Part model, mm, in its own coordinate system. A direction names the side the tool comes from. Give positions to 0.01 mm unless a question says otherwise; leave off trailing zeros. Write each loop counter-clockwise with the first axis right and the second up, starting at its lowest first coordinate (ties: lowest second). Pieces come first, ordered by that corner, then holes. Notation, with made-up numbers: (-36.5, 70) - (-13.5, 70) arc R9 ccw to (-13.5, 74) - close; hole circle Ø9 at (35, 22.5). An arc over 180 degrees is marked (long way). Answer as a JSON object with one key per item and string values. Group by question number.
```python
from build123d import *

# Parameters (mm, degrees)
EXTRUDE_1_DEPTH = 1.68
SKETCH_2_R      = 14.75
EXTRUDE_3_DEPTH = 5


with BuildPart() as part:
    # 草图1 → 凸台-拉伸1 (new body)
    with BuildSketch(Plane(origin=(0, 0, 0), x_dir=(1, 0, 0), z_dir=(0, 1, 0))):
        with BuildLine():
            ThreePointArc((-21.5, 23.6), (-19.6254834, 28.1254834), (-15.1, 30))
            Line((-15.1, 30), (15.1, 30))
            ThreePointArc((15.1, 30), (19.6254834, 28.1254834), (21.5, 23.6))
            Line((21.5, 23.6), (21.5, -23.6))
            ThreePointArc((21.5, -23.6), (19.6254834, -28.1254834), (15.1, -30))
            Line((15.1, -30), (-15.1, -30))
            ThreePointArc((-15.1, -30), (-19.6254834, -28.1254834), (-21.5, -23.6))
            Line((-21.5, -23.6), (-21.5, 23.6))
        make_face()
        with BuildLine():
            ThreePointArc((-18.2, -23.95), (-15, -27.15), (-11.8, -23.95))
            Line((-11.8, -23.95), (-11.8, -21.05))
            ThreePointArc((-11.8, -21.05), (-15, -17.85), (-18.2, -21.05))
            Line((-18.2, -21.05), (-18.2, -23.95))
        make_face(mode=Mode.SUBTRACT)
        with BuildLine():
            ThreePointArc((18.2, -21.05), (15, -17.85), (11.8, -21.05))
            Line((11.8, -21.05), (11.8, -23.95))
            ThreePointArc((11.8, -23.95), (15, -27.15), (18.2, -23.95))
            Line((18.2, -23.95), (18.2, -21.05))
        make_face(mode=Mode.SUBTRACT)
        with BuildLine():
            ThreePointArc((18.2, 23.95), (15, 27.15), (11.8, 23.95))
            Line((11.8, 23.95), (11.8, 21.05))
            ThreePointArc((11.8, 21.05), (15, 17.85), (18.2, 21.05))
            Line((18.2, 21.05), (18.2, 23.95))
        make_face(mode=Mode.SUBTRACT)
        with BuildLine():
            ThreePointArc((-18.2, 21.05), (-15, 17.85), (-11.8, 21.05))
            Line((-11.8, 21.05), (-11.8, 23.95))
            ThreePointArc((-11.8, 23.95), (-15, 27.15), (-18.2, 23.95))
            Line((-18.2, 23.95), (-18.2, 21.05))
        make_face(mode=Mode.SUBTRACT)
    extrude(amount=EXTRUDE_1_DEPTH)

    # 草图2 → 凸台-拉伸3 (add)
    with BuildSketch(Plane(origin=(0, 1.68, 0), x_dir=(1, 0, 0), z_dir=(0, 1, 0))):
        Circle(SKETCH_2_R)
    extrude(amount=EXTRUDE_3_DEPTH)


solid = part.part
```
1) Saw through at D-D (z = 0). List the corners of the cut face in (x, y), and give its area (3 significant figures).
2) Which spindle directions (+Z, -Z, +X, -X, +Y, -Y) get a long thin tool onto all of the face, cutting with end or side? Do faces 1 (the cylindrical face through (14.93, 0.83, -17.85)), 2 (the cylindrical face through (14.07, 4.14, -4.43)), 3 (the flat face through (-21.5, 1, 0)). Say none if no direction does.
3) Saw through at C-C (x = 0). List the corners of the cut face in (y, z).
4) Drill centre lines: line 1 along Z through (x, y) = (-12.5, 1); line 2 along X through (y, z) = (1.5, -19); line 3 along Z through (x, y) = (13.5, 1.5). Where is each one in solid material? Low to high. Write a range as from..to.
5) Two-plate mould, pull along Z, no slides. Class faces 4 (the flat face through (21.5, 1, 0)), 5 (the flat face through (18.2, 1, 23)), 6 (the flat face through (-11.8, 1, -22)), 7 (the cylindrical face through (19.67, 0.83, 28.08)): +Z half, -Z half, draft (parallel to the pull), parting line (faces both ways), or undercut.
6) Saw through at A-A (z = -18.5). List the corners of the cut face in (x, y).
7) Saw through at B-B (x = -13). List the corners of the cut face in (y, z), and give its area (3 significant figures).
Checks:
{
 "1": {"outline": "(-21.5, 0) - (21.5, 0) - (21.5, 1.68) - (14.75, 1.68) - (14.75, 6.68) - (-14.75, 6.68) - (-14.75, 1.68) - (-21.5, 1.68) - close", "area": "220 mm2"},
 "2": {"face 1": "+Y, -Y", "face 2": "+Y", "face 3": "+Z, -Z, -X, +Y, -Y"},
 "3": {"outline": "(0, -30) - (1.68, -30) - (1.68, -14.75) - (6.68, -14.75) - (6.68, 14.75) - (1.68, 14.75) - (1.68, 30) - (0, 30) - close"},
 "4": {"line 1": "-30..-25.95, -19.05..19.05, 25.95..30", "line 2": "-21.5..-17.46, -12.54..12.54, 17.46..21.5", "line 3": "-30..-26.78, -18.22..18.22, 26.78..30"},
 "5": {"face 4": "draft", "face 5": "undercut", "face 6": "undercut", "face 7": "+Z half"},
 "6": {"outline": "(-21.5, 0) - (-16.93, 0) - (-16.93, 1.68) - (-21.5, 1.68) - close; (-13.07, 0) - (13.07, 0) - (13.07, 1.68) - (-13.07, 1.68) - close; (16.93, 0) - (21.5, 0) - (21.5, 1.68) - (16.93, 1.68) - close"},
 "7": {"outline": "(0, -30) - (1.68, -30) - (1.68, -26.45) - (0, -26.45) - close; (0, -18.55) - (1.68, -18.55) - (1.68, -6.97) - (6.68, -6.97) - (6.68, 6.97) - (1.68, 6.97) - (1.68, 18.55) - (0, 18.55) - close; (0, 26.45) - (1.68, 26.45) - (1.68, 30) - (0, 30) - close", "area": "144 mm2"}
}
